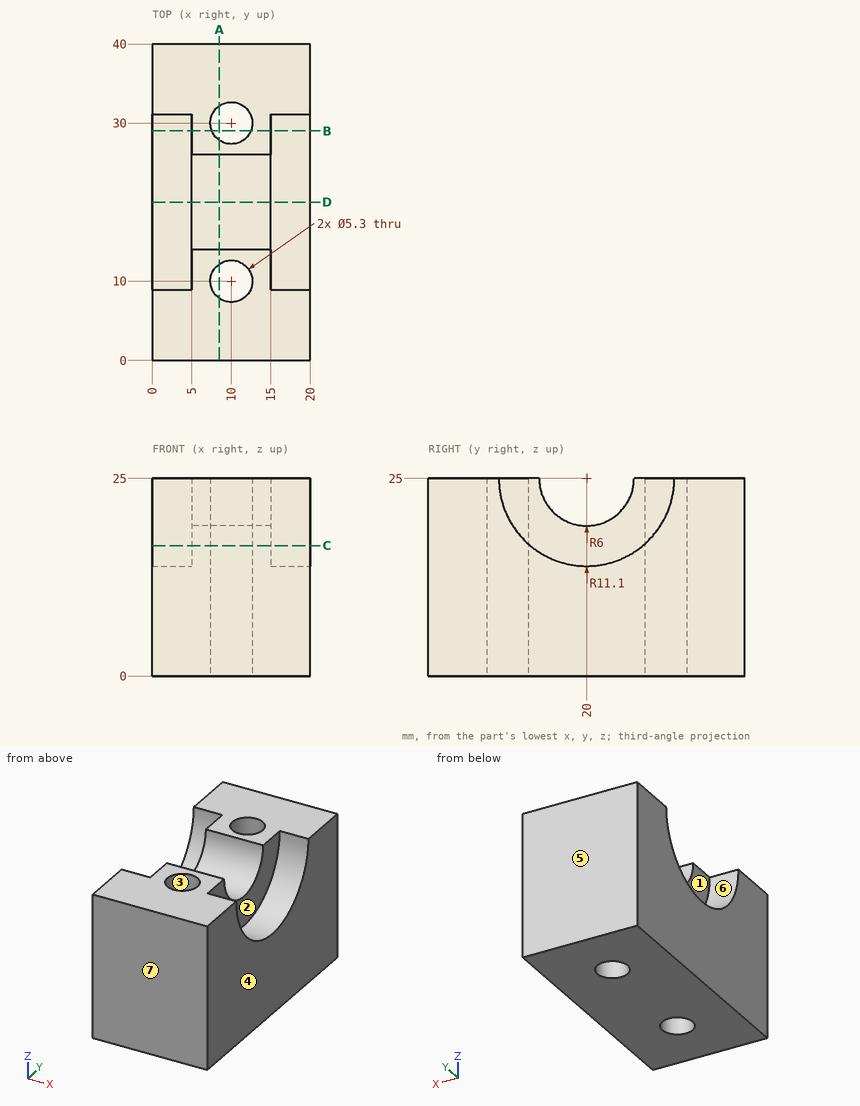
The drawing under review shows one solid part. Ordinate dimensions are in mm from its lowest x, y, z. A direction names the side the tool comes from. Give positions to 0.01 mm unless a question says otherwise; leave off trailing zeros. Loops run counter-clockwise (first coordinate to the right, second up) from the corner with the lowest first, then second, coordinate; pieces in that order, holes last. Notation, with made-up numbers: M -20,66 L -6,66 A16 cw -6,84 Z; hole C 65,-28 d7. An arc over 180 degrees is marked long. One line per item, written item: value. Start each with the question number.
Q1. Clearance check with flat-ended pins moving along their axes: pin 1 Ø9 at (y, z) = (16.5, 20) entering from +X; pin 2 Ø1 at (y, z) = (19, 17) entering from -X. State where each tip first meets the part, or that it passes through.
Q2. Add section D-D (y = 20). Give the boundary of the cut face in (x, z).
Q3. Add section B-B (y = 29). Give the boundary of the cut face in (x, z), and give its area (3 significant figures).
Q4. Machinability: for the marked faces 1, 2 and 3, which of the approach directions +Z, -Z, +X, -X, +Y, -Y give a long, thin tool a straight path to every point of the face, cutting with its end or side? Answer none if there is none.
Q5. Add section C-C (z = 16.5). Give the boundary of the cut face in (x, y), and give its area (3 significant figures).
Q6. Add section A-A (x = 8.5). Give the boundary of the cut face in (y, z), and give its area (3 significant figures).
Q7. Draft analysis for pull direction Y (two halves, no side actions). For the marked faces 4, 5, 6 and 7, state which applies: released by +Y, released by -Y, zero draft, split by the parting line, or undercut.
Q8. For L1, parallel to Y at x = 10, z = 8.25; L2, parallel to X at y = 30, z = 7; L3, parallel to Y at x = 10, z = 20, list the stretches that pass through material, from the lowest coordinate up.
Reply:
1. pin 1: x = 15
1. pin 2: x = 5
2. outline: M 0,0 L 20,0 L 20,13.9 L 15,13.9 L 15,19 L 5,19 L 5,13.9 L 0,13.9 Z
3. outline: M 0,0 L 7.55,0 L 7.55,25 L 5,25 L 5,18.5 L 0,18.5 Z; M 12.45,0 L 20,0 L 20,18.5 L 15,18.5 L 15,25 L 12.45,25 Z
3. area: 312 mm²
4. face 1: +Z, -X
4. face 2: +Z, +X
4. face 3: +Z, -Z
5. outline: M 0,0 L 20,0 L 20,12.86 L 15,12.86 L 15,27.14 L 20,27.14 L 20,40 L 0,40 L 0,27.14 L 5,27.14 L 5,12.86 L 0,12.86 Z; hole C 10,10 d5.3; hole C 10,30 d5.3
5. area: 613 mm²
6. outline: M 0,0 L 7.82,0 L 7.82,25 L 0,25 Z; M 12.18,0 L 27.82,0 L 27.82,25 L 26,25 A6 cw 14,25 L 12.18,25 Z; M 32.18,0 L 40,0 L 40,25 L 32.18,25 Z
6. area: 725 mm²
7. face 4: zero draft
7. face 5: released by +Y
7. face 6: undercut
7. face 7: released by -Y
8. L1: 0 to 7.35, 12.65 to 27.35, 32.65 to 40
8. L2: 0 to 7.35, 12.65 to 20
8. L3: 0 to 7.35, 12.65 to 16.68, 23.32 to 27.35, 32.65 to 40
